```python
from build123d import *

# Parameters (mm, degrees)
ESQUISSE1_W             = 20
ESQUISSE1_H             = 20
BOSS_EXTRU_1_DEPTH      = 5
ESQUISSE2_W             = 5
ESQUISSE2_H             = 5
ENL_V_MAT_EXTRU_1_DEPTH = 5


with BuildPart() as part:
    # Esquisse1 → Boss.-Extru.1 (new body)
    with BuildSketch(Plane.XY):
        with Locations((-33.243041797, 4.26352657)):
            Rectangle(ESQUISSE1_W, ESQUISSE1_H)
    extrude(amount=BOSS_EXTRU_1_DEPTH)

    # Esquisse2 → Enlèv. mat.-Extru.1 (cut)
    with BuildSketch(Plane.XY.offset(5)):
        with Locations((-30.743041797, -3.23647343)):
            Rectangle(ESQUISSE2_W, ESQUISSE2_H)
        with Locations((-40.743041797, -3.23647343)):
            Rectangle(ESQUISSE2_W, ESQUISSE2_H)
        with Locations((-40.743041797, 6.76352657)):
            Rectangle(ESQUISSE2_W, ESQUISSE2_H)
        Polygon((-23.243041797, 14.26352657), (-38.243041797, 14.26352657), (-23.243041797, -0.73647343), align=None)
    extrude(amount=-ENL_V_MAT_EXTRU_1_DEPTH, mode=Mode.SUBTRACT)


solid = part.part
```
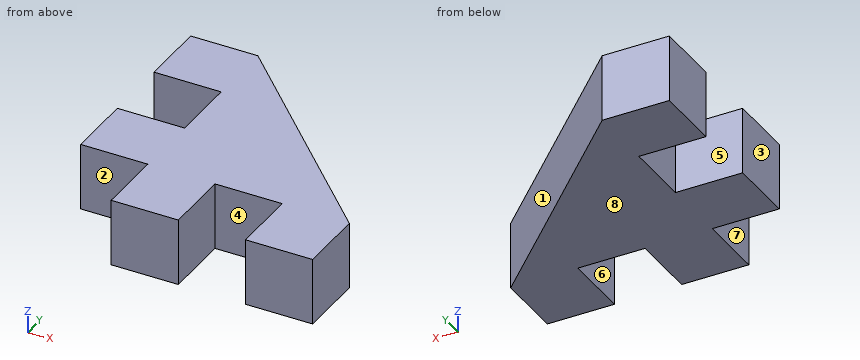
Can you work these out from the model? Positions are in its coordinate system, mm. Face numbers are marked on the shaded views. A direction names the side the tool comes from. Round coordinates to 2 decimals unless told otherwise and drop trailing zeros. Loops run counter-clockwise (first coordinate to the right, second up) from the corner with the lowest first, then second, coordinate; pieces in that order, holes last. Notation, with made-up numbers: M -18.75,-5.75 L 32.25,-5.75 A33 cw 32.25,23.25 Z; hole C 21.5,26 d11. An arc over 180 degrees is marked long. Answer as a JSON object with one key per item and string values. Group by question number.
Q1. We'd pull the mould along X, two halves only. Please class the marked faces 1, 2, 3 and 4: +X half, -X half, draft (parallel to the pull), parting line (faces both ways), or undercut.
Q2. Imagine slicing it at B-B, the plane x = -41.75. Please give me the cut outline in (y, z), then the cut area to 3 significant figures.
Q3. Imagine slicing it at C-C, the plane z = 0.3. Please give me the cut outline in (x, y), then the cut area to 4 significant figures.
Q4. Please list where these lines run through material, in increasing order: L1, parallel to X at y = -1, z = 4.25; L2, parallel to Y at x = -38.5, z = 2.4; L3, parallel to Y at x = -36.25, z = 0.9.
Q5. Imagine slicing it at D-D, the plane y = 11. Please give me the cut outline in (x, z), then the cut area to 3 significant figures.
Q6. On a 3-axis mill with a long thin cutter (end or side, diameter ignored), from which of +Z, -Z, +X, -X, +Y, -Y can I reach the whole of each face in a straight line? I mean the marked faces 5, 6, 7 and 8. Say none if no direction works.
Q7. Imagine slicing it at A-A, the plane y = -3.5. Please give me the cut outline in (x, z), then the cut area to 3 significant figures.
Q8. Will these pins go through, and if not, where does the flat tip stop? pin 1 (2 mm diameter, centred on x = -40, y = 6.5, fed in from +Z); pin 2 (1.5 mm diameter, centred on y = -3.5, z = 2.5, fed in from -X); pin 3 (2.5 mm diameter, centred on x = -31.5, z = 3, fed in from -Y).
Findings:
{
 "1": {"face 1": "+X half", "face 2": "draft", "face 3": "-X half", "face 4": "undercut"},
 "2": {"outline": "M -0.74,0 L 4.26,0 L 4.26,5 L -0.74,5 Z; M 9.26,0 L 14.26,0 L 14.26,5 L 9.26,5 Z", "area": "50.0 mm2"},
 "3": {"outline": "M -43.24,-0.74 L -38.24,-0.74 L -38.24,-5.74 L -33.24,-5.74 L -33.24,-0.74 L -28.24,-0.74 L -28.24,-5.74 L -23.24,-5.74 L -23.24,-0.74 L -38.24,14.26 L -43.24,14.26 L -43.24,9.26 L -38.24,9.26 L -38.24,4.26 L -43.24,4.26 Z", "area": "212.5 mm2"},
 "4": {"L1": "x = -38.24 to -33.24, -28.24 to -23.24", "L2": "y = -0.74 to 4.26, 9.26 to 14.26", "L3": "y = -5.74 to 12.27"},
 "5": {"outline": "M -43.24,0 L -34.98,0 L -34.98,5 L -43.24,5 Z", "area": "41.3 mm2"},
 "6": {"face 5": "+Z, -Z, -X", "face 6": "+Z, -Z, -Y", "face 7": "+Z, -Z, -X, -Y", "face 8": "-Z, +X, -X, +Y, -Y"},
 "7": {"outline": "M -38.24,0 L -33.24,0 L -33.24,5 L -38.24,5 Z; M -28.24,0 L -23.24,0 L -23.24,5 L -28.24,5 Z", "area": "50.0 mm2"},
 "8": {"pin 1": "passes through", "pin 2": "stops at x = -38.24", "pin 3": "stops at y = -0.74"}
}
